Autodesk Inventor part; units mm, degrees
ref_plane "YZ Plane" through (0, 0, 0) normal (1, 0, 0) x (0, 1, 0)
ref_plane "XZ Plane" through (0, 0, 0) normal (0, 1, 0) x (-1, 0, 0)
ref_plane "XY Plane" through (0, 0, 0) normal (0, 0, 1) x (1, 0, 0)
sketch "Sketch1" plane through (0, 0, 0) normal (0, 1, 0) x (-1, 0, 0)
  line L0 (0, 0) -> (-80, 0)
  line L1 (-80, 0) -> (-80, -34)
  line L2 (-80, -34) -> (0, -34)
  line L3 (0, -34) -> (0, 0)
  dimension "d0" = 80
  dimension "d1" = 34
extrude "Extrusion1" add sketch "Sketch1" along normal blind 36
sketch "Sketch2" plane through (80, 0, 0) normal (1, 0, 0) x (0, 0, -1)
  line L0 (0, 0) -> (34, 0)
  line L1 (34, 0) -> (34, 36)
  line L2 (0, 36) -> (34, 36)
  line L3 (0, 0) -> (0, 36)
  line L4 (0, 0) -> (10, 0)
  line L5 (10, 0) -> (10, 31)
  line L6 (10, 31) -> (0, 31)
  line L7 (0, 31) -> (0, 0)
  dimension "d4" = 5
  dimension "d5" = 24
extrude "Extrusion2" cut sketch "Sketch2" against normal through all contours L3 L6 L5 L0
properties part number "cushion"
Can you work these out from the model? Positions are in its coordinate system, mm. A direction names the side the tool comes from. Coordinates: 2 decimals unless noted, no trailing zeros. Order: outer loops, then holes, each group sorted by start corner. A loop starts at its lowest first (then second) coordinate and runs counter-clockwise, first axis right, second up. Notation, with made-up numbers: M -28,37 L 14,37 A18 ccw 14,56 Z; hole C 75.25,3.5 d3. An arc over 180 degrees is marked long. Write item = value, one per line.
(1) Suppose I cut it at B-B on y = 9.5. Please give me the cut outline in (x, z), plus the area to 3 significant figures.
Results are:
outline = M 0,-34 L 80,-34 L 80,-10 L 0,-10 Z
area = 1,920 mm2
(2) If we mould it in two halves opening along X, with no side actions, what happens to faces 1 (the face through (0, 18, -21)), 2 (the face through (80, 18, -21)), 3 (the face through (41, 36, -17))? For each: pulls with the +X half, pulls with the -X half, needs draft (parallel to the pull), parting line crosses it, or undercut.
Results are:
face_1 = pulls with the -X half
face_2 = pulls with the +X half
face_3 = needs draft
(3) For faces 4 (the face through (41, 15, -10)), 5 (the face through (41, 18, -34)), which set-ups out of +Z, -Z, +X, -X, +Y, -Y let a thin tool reach every point of the face, with its end or its side?
Results are:
face_4 = +Z, +X, -X, -Y
face_5 = -Z, +X, -X, +Y, -Y
(4) For pin 1 Ø4 at (y, z) = (30.5, -3.5) entering from -X; pin 2 Ø2 at (x, y) = (18, 25.5) entering from +Z, each with a flat end and sliding along its axis, tell me the tip position at first contact or that it passes through.
Results are:
pin_1 = 0
pin_2 = -10
(5) I need wall thicknesses on line 1 along Y through (x, z) = (24, -6); line 2 along Z through (x, y) = (54.5, 23). Which ranges of each line are inside material? Lowest first, please. Write a range as [from, to].
Results are:
line_1 = [31, 36]
line_2 = [-34, -10]
(6) Suppose I cut it at C-C on z = -3. Please give me the cut outline in (x, y).
Results are:
outline = M 0,31 L 80,31 L 80,36 L 0,36 Z
(7) Suppose I cut it at A-A on x = 45. Please give me the cut outline in (y, z), plus the area to 3 significant figures.
Results are:
outline = M 0,-34 L 36,-34 L 36,0 L 31,0 L 31,-10 L 0,-10 Z
area = 914 mm2
